from build123d import *

# Parameters (mm, degrees)
SKETCH_1_R          = 15
EXTRUDE_1_DEPTH     = 4
SKETCH_2_W          = 10
SKETCH_2_H          = 3
EXTRUDE_2_DEPTH     = 12
SKETCH_3_R          = 2.1
CUT_EXTRUDE_1_DEPTH = 16


with BuildPart() as part:
    # 草图1 → 凸台-拉伸1 (new body)
    with BuildSketch(Plane.XY):
        Circle(SKETCH_1_R)
    extrude(amount=EXTRUDE_1_DEPTH)

    # 草图2 → 凸台-拉伸2 (add)
    with BuildSketch(Plane.XY):
        with Locations((0, -4.6)):
            Rectangle(SKETCH_2_W, SKETCH_2_H)
        with Locations((0, 4.6)):
            Rectangle(SKETCH_2_W, SKETCH_2_H)
    extrude(amount=-EXTRUDE_2_DEPTH)

    # 草图3 → 切除-拉伸1 (cut)
    with BuildSketch(Plane(origin=(0, 6.1, 0), x_dir=(1, 0, 0), z_dir=(0, 1, 0))):
        with Locations(Location((0, 7, 0), (0, 0, 270))):
            Circle(SKETCH_3_R)
    extrude(amount=-CUT_EXTRUDE_1_DEPTH, mode=Mode.SUBTRACT)


solid = part.part
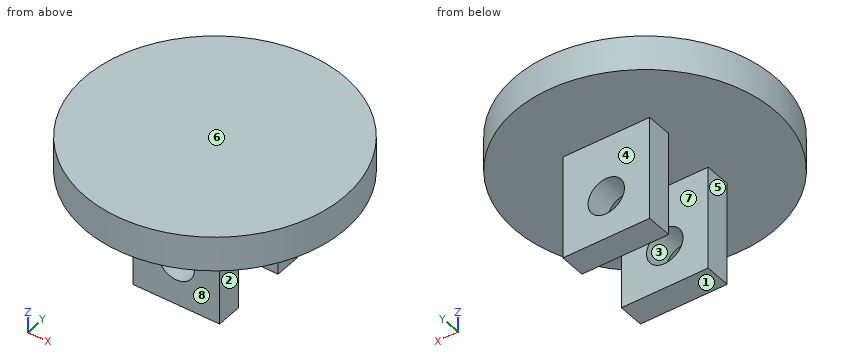
Here's how the part is built. I have some questions about the finished solid (model axes, mm). Face numbers are marked on the shaded views. A direction names the side the tool comes from. Round coordinates to 2 decimals unless told otherwise and drop trailing zeros. Loops run counter-clockwise (first coordinate to the right, second up) from the corner with the lowest first, then second, coordinate; pieces in that order, holes last. Notation, with made-up numbers: M 60,-31.75 L 96,-31.75 A23 cw 96,2.25 Z; hole C 17,82.5 d3. An arc over 180 degrees is marked long. Write each question's results on one line, items separated by ' | '. Start each with the question number.
(1) I want a section at A-A (z = -3). Please give me the cut outline in (x, y).
(2) Will these pins go through, and if not, where does the flat tip stop? P1, Ø8, axis at y = -12, z = 0, coming from the -X side; P2, Ø10, axis at x = -3, y = 10, coming from the -Z side; P3, Ø8, axis at x = 0.5, z = -5, coming from the -Y side; P4, Ø8, axis at x = -8.5, z = -3, coming from the +Y side.
(3) I want a section at C-C (x = 3). Please give me the cut outline in (y, z).
(4) On a 3-axis mill with a long thin cutter (end or side, diameter ignored), from which of +Z, -Z, +X, -X, +Y, -Y can I reach the whole of each face in a straight line? I mean the marked faces 4, 5, 6, 7 and 8. Say none if no direction works.
(5) Thinking about a two-plate mould opening in Z: for the marked faces 1, 2 and 3, which applies, pulls with the +Z half, pulls with the -Z half, needs draft (parallel to the pull), parting line crosses it, or undercut?
(6) I want a section at D-D (y = 12). Please give me the cut outline in (x, z).
(7) If I drill on probe 1 along X at (y, z) = (5.1, -7); probe 2 along Y at (x, z) = (4.25, -0.5); probe 3 along Z at (x, y) = (-7.25, -10.5), over which ranges is the centre line in solid material (lowest first)? Write a range as from..to.
(8) I want a section at B-B (z = -7). Please give me the cut outline in (x, y).
Solved:
1) outline: M -5,-6.1 L 5,-6.1 L 5,-3.1 L -5,-3.1 Z; M -5,3.1 L 5,3.1 L 5,6.1 L -5,6.1 Z
2) P1: stops at x = -12.69 | P2: stops at z = -12 | P3: stops at y = -6.1 | P4: stops at y = 13.81
3) outline: M -14.7,0 L -6.1,0 L -6.1,-12 L -3.1,-12 L -3.1,0 L 3.1,0 L 3.1,-12 L 6.1,-12 L 6.1,0 L 14.7,0 L 14.7,4 L -14.7,4 Z
4) face 4: -Z, +X, -X, +Y | face 5: -Z, -X, +Y, -Y | face 6: +Z, +X, -X, +Y, -Y | face 7: -Z, +X, -X | face 8: -Z, +X, -X, -Y
5) face 1: pulls with the -Z half | face 2: needs draft | face 3: undercut
6) outline: M -9,0 L 9,0 L 9,4 L -9,4 Z
7) probe 1: x = -5..-2.1, 2.1..5 | probe 2: y = -6.1..-3.1, 3.1..6.1 | probe 3: z = 0..4
8) outline: M -5,-6.1 L -2.1,-6.1 L -2.1,-3.1 L -5,-3.1 Z; M -5,3.1 L -2.1,3.1 L -2.1,6.1 L -5,6.1 Z; M 2.1,-6.1 L 5,-6.1 L 5,-3.1 L 2.1,-3.1 Z; M 2.1,3.1 L 5,3.1 L 5,6.1 L 2.1,6.1 Z
